Geometry: final body of the model. Coordinates: model frame, mm. Give positions to 0.01 mm unless a question says otherwise; leave off trailing zeros. Write each loop counter-clockwise with the first axis right and the second up, starting at its lowest first coordinate (ties: lowest second). Pieces come first, ordered by that corner, then holes. Notation, with made-up numbers: M -11.75,-3 L 33.25,-3 A20 cw 33.25,24 Z; hole C -24,45 d4. An arc over 180 degrees is marked long. Answer as a JSON object with one key per item and string values.
from build123d import *

# Parameters (mm, degrees)
BOSS_EXTRUDE1_DEPTH = 3
SKETCH3_W           = 27
SKETCH3_H           = 5
BOSS_EXTRUDE2_DEPTH = 3
SKETCH4_W           = 8
SKETCH4_H           = 3
CUT_EXTRUDE1_DEPTH  = 3
SKETCH5_W           = 5
SKETCH5_H           = 3.9
CUT_EXTRUDE2_DEPTH  = 3
SKETCH6_W           = 5
SKETCH6_H           = 4.739085619
CUT_EXTRUDE3_DEPTH  = 3
SKETCH7_W           = 7
SKETCH7_H           = 3
CUT_EXTRUDE5_DEPTH  = 3
SKETCH8_W           = 4.245961236
SKETCH8_H           = 1.503952676
CUT_EXTRUDE6_DEPTH  = 10


# Read off the part's stored shape, not the designer's step: Boss-Extrude1
with BuildPart() as part:
    # Boss-Extrude1 outline → Boss-Extrude1 (new body)
    with BuildSketch(Plane.XY):
        Polygon((195, -43.4), (200, -43.4), (200, -16.4), (195, -16.4), (195, -13.4), (200, -13.4), (200, 13.6), (195, 13.6), (195, 16.6), (200, 16.6), (200, 43.6), (195, 43.6), (195, 47.5), (190, 47.5), (190, 52.5), (163, 52.5), (163, 47.5), (119.4, 47.5), (119.4, 52.5), (92.4, 52.5), (92.4, 47.5), (48.8, 47.5), (48.8, 52.5), (21.8, 52.5), (21.8, 47.5), (-21.8, 47.5), (-21.8, 52.5), (-48.8, 52.5), (-48.8, 47.5), (-92.4, 47.5), (-92.4, 52.5), (-119.4, 52.5), (-119.4, 47.5), (-163, 47.5), (-163, 52.5), (-190, 52.5), (-190, 47.5), (-189.5, 47.5), (-189.5, 43.6), (-200, 43.6), (-200, 16.6), (-187, 16.6), (-187, 13.6), (-200, 13.6), (-200, -13.4), (-187, -13.4), (-187, -16.4), (-200, -16.4), (-200, -43.4), (-187, -43.4), (-187, -47.5), (195, -47.5), align=None)
    extrude(amount=BOSS_EXTRUDE1_DEPTH)

    # Sketch3 → Boss-Extrude2 (add)
    with BuildSketch(Plane.XY.offset(3)):
        with Locations((-176.5, -50)):
            Rectangle(SKETCH3_W, SKETCH3_H)
        with Locations((-105.9, -50)):
            Rectangle(SKETCH3_W, SKETCH3_H)
        with Locations((-35.3, -50)):
            Rectangle(SKETCH3_W, SKETCH3_H)
        with Locations((35.3, -50)):
            Rectangle(SKETCH3_W, SKETCH3_H)
        with Locations((105.9, -50)):
            Rectangle(SKETCH3_W, SKETCH3_H)
        with Locations((176.5, -50)):
            Rectangle(SKETCH3_W, SKETCH3_H)
    extrude(amount=-BOSS_EXTRUDE2_DEPTH)

    # Sketch4 → Cut-Extrude1 (cut)
    with BuildSketch(Plane.XY.offset(3)):
        with Locations((191, -14.9)):
            Rectangle(SKETCH4_W, SKETCH4_H)
        with Locations((191, 15.1)):
            Rectangle(SKETCH4_W, SKETCH4_H)
        with Locations((191, -44.9)):
            Rectangle(SKETCH4_W, SKETCH4_H)
    extrude(amount=-CUT_EXTRUDE1_DEPTH, mode=Mode.SUBTRACT)

    # Sketch5 → Cut-Extrude2 (cut)
    with BuildSketch(Plane.XY.offset(3)):
        with Locations((192.5, 45.55)):
            Rectangle(SKETCH5_W, SKETCH5_H)
    extrude(amount=-CUT_EXTRUDE2_DEPTH, mode=Mode.SUBTRACT)

    # Sketch6 → Cut-Extrude3 (cut)
    with BuildSketch(Plane.XY.offset(3)):
        with Locations((192.522405585, -47.571722604)):
            Rectangle(SKETCH6_W, SKETCH6_H)
    extrude(amount=-CUT_EXTRUDE3_DEPTH, mode=Mode.SUBTRACT)

    # Sketch7 → Cut-Extrude5 (cut)
    with BuildSketch(Plane.XY.offset(3)):
        with Locations((186.5, -47.902198406)):
            Rectangle(SKETCH7_W, SKETCH7_H)
    extrude(amount=-CUT_EXTRUDE5_DEPTH, mode=Mode.SUBTRACT)

    # Sketch8 → Cut-Extrude6 (cut)
    with BuildSketch(Plane.XY.offset(3)):
        with Locations((189.30979268, -47.154174744)):
            Rectangle(SKETCH8_W, SKETCH8_H)
    extrude(amount=-CUT_EXTRUDE6_DEPTH, mode=Mode.SUBTRACT)


solid = part.part
1) Contact query for flat-ended pins moving along their axis: P1, Ø0.9, axis at x = -75.5, z = 1, coming from the +Y side; P2, Ø1.5, axis at y = -50.5, z = 2, coming from the -X side; P3, Ø0.9, axis at x = 61.5, z = 1, coming from the -Y side. Output: stop coordinate, or through.
Geometry check:
{"P1": "stops at y = 47.5", "P2": "stops at x = -190", "P3": "stops at y = -47.5"}
2) Cut plane A-A on x = -63.5. Return loops of the section in (y, z), and give its area (3 significant figures).
Geometry check:
{"outline": "M -47.5,0 L 47.5,0 L 47.5,3 L -47.5,3 Z", "area": "285 mm2"}
3) Line query: line 1 (Y direction, x = -69.5, z = 0.65); line 2 (X direction, y = -47, z = 2.8); line 3 (X direction, y = -14, z = 1.2). Output: solid intervals per line, ascending. Write a range as from..to.
Geometry check:
{"line 1": "y = -47.5..47.5", "line 2": "x = -187..183", "line 3": "x = -187..187"}
